Autodesk Inventor part; units mm, degrees
ref_plane "YZ Plane" through (0, 0, 0) normal (1, 0, 0) x (0, 1, 0)
ref_plane "XZ Plane" through (0, 0, 0) normal (0, 1, 0) x (-1, 0, 0)
ref_plane "XY Plane" through (0, 0, 0) normal (0, 0, 1) x (1, 0, 0)
ref_plane "Work Plane1" through (-7.9975, -173.6428, 0) normal (0, 0, 1) x (0.9989, -0.0477, 0)
sketch "Sketch1" plane through (-7.9975, -173.6428, 0) normal (0, 0, 1) x (0.9989, -0.0477, 0)
  circle A0 centre (24.871, 68.4391) radius 19.05
  circle A1 centre (37.9927, 67.6226) radius 1.8542
  circle A2 centre (25.6875, 81.5607) radius 1.8542
  circle A3 centre (11.7494, 69.2555) radius 1.8542
  circle A4 centre (24.0546, 55.3174) radius 1.8542
  circle A5 centre (24.871, 68.4391) radius 3.175
  point P0 (-0.2983, 173.8266)
extrude "Extrusion1" add sketch "Sketch1" against normal blind 6.35
properties part number "gearGuideDiscOutputStage1"
Geometry check sheet. Reference: the model listing, model coordinates, mm. Coordinates: 2 decimals unless noted, no trailing zeros. Order: outer loops, then holes, each group sorted by start corner. A loop starts at its lowest first (then second) coordinate and runs counter-clockwise, first axis right, second up. Notation, with made-up numbers: M 53.5,-13.75 L 63.5,-13.75 A38 cw 63.5,24.25 Z; hole C 46.5,22.25 d10. An arc over 180 degrees is marked long. Answer as a JSON object with one key per item and string values.
Q1. Release check for a two-part mould opening along Y. For faces 1 (the cylindrical face through (34.854, -108.7, -3.131)), 2 (the cylindrical face through (15.098, -124.847, -3.131)), 3 (the flat face through (20, -110, -6.35)) record: released by +Y, released by -Y, zero draft, split by the parting line, or undercut.
Results are:
{"face 1": "undercut", "face 2": "split by the parting line", "face 3": "zero draft"}
Q2. Cross-section at B-B on y = -108.5. Record the cut outline in (x, z), and give its area (3 significant figures).
Results are:
{"outline": "M 1.17,-6.35 L 17.67,-6.35 L 17.67,0 L 1.17,0 Z; M 22.55,-6.35 L 31.42,-6.35 L 31.42,0 L 22.55,0 Z; M 34.94,-6.35 L 39.05,-6.35 L 39.05,0 L 34.94,0 Z", "area": "187 mm²"}
Q3. Cross-section at C-C on x = 33.5. Record the cut outline in (y, z), and give its area (3 significant figures).
Results are:
{"outline": "M -120.02,-6.35 L -109.74,-6.35 L -109.74,0 L -120.02,0 Z; M -106.08,-6.35 L -92.92,-6.35 L -92.92,0 L -106.08,0 Z", "area": "149 mm²"}
Q4. Scan lines: line 1 (Y direction, x = 19, z = -1.75); line 2 (X direction, y = -108, z = -5.5); line 3 (X direction, y = -105.5, z = -2.5) (3 decimals). Record each from-to range of solid material in increasing order.
Results are:
{"line 1": "y = -125.49 to -121.36, -117.71 to -109.44, -103.49 to -87.45", "line 2": "x = 1.12 to 17.33, 22.89 to 31.33, 35.03 to 39.1", "line 3": "x = 1.084 to 5.249, 8.835 to 17.086, 23.133 to 39.135"}
Q5. Cross-section at A-A on x = 7. Record the cut outline in (y, z).
Results are:
{"outline": "M -120.29,-6.35 L -106.88,-6.35 L -106.88,0 L -120.29,0 Z; M -103.17,-6.35 L -92.65,-6.35 L -92.65,0 L -103.17,0 Z"}
Q6. Depth check by flat-ended pin: pin 1 Ø3 at (x, y) = (7.04, -105.03) entering from +Z; pin 2 Ø4.5 at (x, y) = (18.67, -119.54) entering from -Z; pin 3 Ø1 at (y, z) = (-113.5, -2) entering from -X. Enter the tip coordinate at first touch or a pass-through.
Results are:
{"pin 1": "passes through", "pin 2": "stops at z = -6.35", "pin 3": "stops at x = 2.21"}
Q7. Cross-section at D-D on x = 11.5. Record the cut outline in (y, z).
Results are:
{"outline": "M -123.46,-6.35 L -89.47,-6.35 L -89.47,0 L -123.46,0 Z"}
